from build123d import *

# Parameters (mm, degrees)
SKETCH1_R           = 17.5
SKETCH1_R_2         = 1.45
BOSS_EXTRUDE1_DEPTH = 5
BOSS_EXTRUDE2_DEPTH = 6.25
CUT_EXTRUDE1_DEPTH  = 7
CUT_EXTRUDE2_DEPTH  = 5.85
BOSS_EXTRUDE3_START = 2
SKETCH5_W           = 6.504597346
SKETCH5_H           = 6.25
SKETCH5_R           = 1.7
BOSS_EXTRUDE3_DEPTH = 2
SKETCH6_R           = 3
CUT_EXTRUDE3_DEPTH  = 1.5
BOSS_EXTRUDE4_START = 1.5
SKETCH7_W           = 6.508151024
SKETCH7_H           = 6.25
SKETCH7_R           = 3
BOSS_EXTRUDE4_DEPTH = 1.5
BOSS_EXTRUDE5_START = -6.25
BOSS_EXTRUDE5_DEPTH = 6.25
BOSS_EXTRUDE6_DEPTH = 1


with BuildPart() as part:
    # Sketch1 → Boss-Extrude1 (new body)
    with BuildSketch(Plane.XZ.offset(-15)):
        with Locations(Location((0, 0, 0), (0, 0, 270))):
            Circle(SKETCH1_R)
        with Locations(Location((-6.234624063, -11.064332912, 0), (0, 0, 270))):
            Circle(SKETCH1_R_2, mode=Mode.SUBTRACT)
        with Locations(Location((11.064332912, -6.234624063, 0), (0, 0, 270))):
            Circle(SKETCH1_R_2, mode=Mode.SUBTRACT)
        with Locations(Location((-11.064332912, 6.234624063, 0), (0, 0, 270))):
            Circle(SKETCH1_R_2, mode=Mode.SUBTRACT)
        with BuildLine():
            ThreePointArc((2.481687642, -1.063591298), (-2.638702415, -0.572057308), (1.818419998, 1.995832837))
            Line((1.818419998, 1.995832837), (1.856473873, 1.82030348))
            Line((1.856473873, 1.82030348), (2.443633767, -0.888061941))
            Line((2.443633767, -0.888061941), (2.481687642, -1.063591298))
        make_face(mode=Mode.SUBTRACT)
        with Locations(Location((6.234624063, 11.064332912, 0), (0, 0, 270))):
            Circle(SKETCH1_R_2, mode=Mode.SUBTRACT)
    extrude(amount=BOSS_EXTRUDE1_DEPTH)

    # Sketch2 → Boss-Extrude2 (add)
    with BuildSketch(Plane.XZ.offset(-10)):
        with BuildLine():
            Line((6.747748589, -1.862226887), (6.059242583, 1.313613078))
            Line((6.059242583, 1.313613078), (5.370736577, 4.489453042))
            ThreePointArc((5.370736577, 4.489453042), (-5.837040783, 3.863800576), (-2.034603986, -6.697789682))
            ThreePointArc((-2.034603986, -6.697789682), (-1.550245392, -6.826180427), (-1.05794298, -6.919592232))
            ThreePointArc((-1.05794298, -6.919592232), (1.483111539, -6.841080336), (3.828542975, -5.860226846))
            ThreePointArc((3.828542975, -5.860226846), (4.323739448, -5.505022905), (4.786164678, -5.108094329))
            ThreePointArc((4.786164678, -5.108094329), (5.990968426, -3.620538264), (6.747748589, -1.862226887))
        make_face()
        with BuildLine():
            ThreePointArc((2.481687642, -1.063591298), (-2.638702415, -0.572057308), (1.818419998, 1.995832837))
            Line((1.818419998, 1.995832837), (2.481687642, -1.063591298))
        make_face(mode=Mode.SUBTRACT)
    extrude(amount=BOSS_EXTRUDE2_DEPTH)

    # Sketch3 → Cut-Extrude1 (cut)
    with BuildSketch(Plane(origin=(6.059242583, 0, 1.313613078), x_dir=(0.21187307702941563, 0, -0.9772971908432395), z_dir=(0.9772971908432395, 0, 0.21187307702941563))):
        with BuildLine():
            ThreePointArc((0, 8.575), (-1.7, 6.875), (0, 5.175))
            Line((0, 5.175), (0, 8.575))
        make_face()
        with BuildLine():
            Line((0, 8.575), (0, 5.175))
            ThreePointArc((0, 5.175), (1.202081528, 5.672918472), (1.7, 6.875))
            ThreePointArc((1.7, 6.875), (1.202081528, 8.077081528), (0, 8.575))
        make_face()
    extrude(amount=-CUT_EXTRUDE1_DEPTH, mode=Mode.SUBTRACT)

    # Sketch4 → Cut-Extrude2 (cut)
    with BuildSketch(Plane.XZ.offset(-3.75)):
        Polygon((3.620479073, -2.540596639), (4.793235702, -2.286348947), (6.161451769, -1.989726639), (4.784276768, 4.362705102), (2.243304072, 3.811835101), align=None)
    extrude(amount=-CUT_EXTRUDE2_DEPTH, mode=Mode.SUBTRACT)

    # Sketch5 → Boss-Extrude3 (add)
    with BuildSketch(Plane(origin=(6.059242583, 0, 1.313613078), x_dir=(0.21187307702941563, 0, -0.9772971908432395), z_dir=(0.9772971908432395, 0, 0.21187307702941563)).offset(BOSS_EXTRUDE3_START)):
        with Locations((-0.002683311, 6.875)):
            Rectangle(SKETCH5_W, SKETCH5_H)
        with Locations((0, 6.875)):
            Circle(SKETCH5_R, mode=Mode.SUBTRACT)
    extrude(amount=-BOSS_EXTRUDE3_DEPTH)

    # Sketch6 → Cut-Extrude3 (cut)
    with BuildSketch(Plane(origin=(8.013836965, 0, 1.737359232), x_dir=(0.21187307702941569, 0, -0.9772971908432395), z_dir=(0.9772971908432395, 0, 0.21187307702941569))):
        with Locations((0, 6.875)):
            Circle(SKETCH6_R)
    extrude(amount=-CUT_EXTRUDE3_DEPTH, mode=Mode.SUBTRACT)

    # Sketch7 → Boss-Extrude4 (add)
    with BuildSketch(Plane(origin=(8.013836965, 0, 1.737359232), x_dir=(0.21187307702941569, 0, -0.9772971908432395), z_dir=(0.9772971908432395, 0, 0.21187307702941569)).offset(BOSS_EXTRUDE4_START)):
        with Locations((-0.00446015, 6.875)):
            Rectangle(SKETCH7_W, SKETCH7_H)
        with Locations((0, 6.875)):
            Circle(SKETCH7_R, mode=Mode.SUBTRACT)
    extrude(amount=-BOSS_EXTRUDE4_DEPTH)

    # Sketch8 → Boss-Extrude5 (add)
    with BuildSketch(Plane.XZ.offset(-3.75).offset(BOSS_EXTRUDE5_START)):
        with BuildLine():
            Line((8.789386774, 5.239726596), (8.577513697, 6.217023787))
            Line((8.577513697, 6.217023787), (0.69957596, 6.964954664))
            ThreePointArc((0.69957596, 6.964954664), (3.27783475, 6.185127271), (5.370736577, 4.489453042))
            Line((5.370736577, 4.489453042), (5.369599535, 4.494697826))
            Line((5.369599535, 4.494697826), (7.324193916, 4.91844398))
            Line((7.324193916, 4.91844398), (7.323440988, 4.921916981))
            Line((7.323440988, 4.921916981), (8.789386774, 5.239726596))
        make_face()
        with BuildLine():
            ThreePointArc((6.747748589, -1.862226887), (5.549511662, -4.266488053), (3.533996626, -6.042422349))
            Line((3.533996626, -6.042422349), (10.380161834, -2.097968308))
            Line((10.380161834, -2.097968308), (10.168288757, -1.120671117))
            Line((10.168288757, -1.120671117), (6.747748589, -1.862226887))
        make_face()
    extrude(amount=BOSS_EXTRUDE5_DEPTH)

    # Sketch10 → Boss-Extrude6 (add)
    with BuildSketch(Plane.XZ.offset(-3.75)):
        with BuildLine():
            Line((8.577513697, 6.217023787), (0.69957596, 6.964954664))
            ThreePointArc((0.69957596, 6.964954664), (-6.839499134, -1.490386391), (3.533996626, -6.042422349))
            Line((3.533996626, -6.042422349), (10.380161834, -2.097968308))
            Line((10.380161834, -2.097968308), (8.577513697, 6.217023787))
        make_face()
        Polygon((6.161451769, -1.989726639), (3.620479073, -2.540596639), (2.243304072, 3.811835101), (4.784276768, 4.362705102), align=None, mode=Mode.SUBTRACT)
        with BuildLine():
            Line((1.818419998, 1.995832837), (2.481687642, -1.063591298))
            ThreePointArc((2.481687642, -1.063591298), (-2.638702415, -0.572057308), (1.818419998, 1.995832837))
        make_face(mode=Mode.SUBTRACT)
    extrude(amount=BOSS_EXTRUDE6_DEPTH)


solid = part.part
Can you work these out from the model? Positions are in its coordinate system, mm. A direction names the side the tool comes from. Coordinates: 2 decimals unless noted, no trailing zeros. Write each loop counter-clockwise with the first axis right and the second up, starting at its lowest first coordinate (ties: lowest second). Pieces come first, ordered by that corner, then holes. Notation, with made-up numbers: (47.5, 4.25) -> (89.5, 4.25) arc R26 ccw to (89.5, 36.25) -> close; hole circle Ø9 at (5.5, -21.5). An arc over 180 degrees is marked (long way). Write each question's results on one line, items separated by ' | '. Start each with the question number.
Item 1: Thinking about a two-plate mould opening in Z: for faces 1 (the flat face through (2, 2.75, 3)), 2 (the flat face through (3.496, 6.223, 4.083)), 3 (the flat face through (4.694, 6.426, 6.586)), 4 (the flat face through (6.909, 6.426, -4.098)), which applies, released by +Z, released by -Z, zero draft, split by the parting line, or undercut?
Item 2: If we section it at D-D, the plane x = -5.5: Write out the boundary of the cut face in (y, z), and give its area (3 significant figures).
Item 3: If we section it at C-C, the plane y = 14.25: Write out the boundary of the cut face in (x, z), and give its area (3 significant figures).
Item 4: I'm going to push flat-ended pins straight in: P1, Ø4, axis at y = 13.5, z = -3, coming from the +X side; P2, Ø3, axis at x = 0.5, y = 6.5, coming from the -Z side; P3, Ø4, axis at x = -7.5, z = -8, coming from the -Y side. Where does each tip first touch, or does it pass through?
Item 5: Please list where these lines run through material, in increasing order: probe 1 along Y at (x, z) = (13, -1.5); probe 2 along Z at (x, y) = (-12, 10.5); probe 3 along Z at (x, y) = (-5.5, 10.5).
Item 6: On a 3-axis mill with a long thin cutter (end or side, diameter ignored), from which of +Z, -Z, +X, -X, +Y, -Y can I reach the whole of each face in a straight line? I mean faces 5 (the flat face through (2.145, 4.12, 0.488)), 6 (the flat face through (5.463, 4.701, 1.231)), 7 (the flat face through (6.54, 4.92, 1.46)). Say none if no direction works.
Item 7: If we section it at B-B, the plane z = 10.5: Write out the boundary of the cut face in (x, y), and give its area (3 significant figures).
Item 8: If we section it at A-A, the plane x = 0: Write out the boundary of the cut face in (y, z).
Answer block:
1) face 1: zero draft | face 2: undercut | face 3: released by +Z | face 4: released by -Z
2) outline: (2.75, -4.33) -> (10, -4.33) -> (10, -9.81) -> (15, -9.81) -> (15, 16.61) -> (10, 16.61) -> (10, 4.33) -> (2.75, 4.33) -> close; (10, -16.61) -> (15, -16.61) -> (15, -12.31) -> (10, -12.31) -> close | area: 216 mm²
3) outline: circle Ø35 at (0, 0); hole circle Ø2.9 at (-11.06, 6.23); hole circle Ø2.9 at (-6.23, -11.06); hole (1.82, 2) arc R2.7 ccw (long way) to (2.48, -1.06) -> close; hole circle Ø2.9 at (6.23, 11.06); hole circle Ø2.9 at (11.06, -6.23) | area: 914 mm²
4) P1: x = 17.47 | P2: z = -7 | P3: y = 10
5) probe 1: 10 to 15 | probe 2: -12.74 to 5.13, 7.34 to 12.74 | probe 3: -16.61 to -12.31, -9.81 to 16.61
6) face 5: +Y, -Y | face 6: -Y | face 7: none
7) outline: (-14, 10) -> (4.9, 10) -> (4.9, 15) -> (-14, 15) -> close; (7.57, 10) -> (14, 10) -> (14, 15) -> (7.57, 15) -> close | area: 127 mm²
8) outline: (2.75, -7) -> (10, -7) -> (10, -17.5) -> (15, -17.5) -> (15, -2.7) -> (2.75, -2.7) -> close; (2.75, 2.7) -> (15, 2.7) -> (15, 17.5) -> (10, 17.5) -> (10, 7) -> (2.75, 7) -> close
